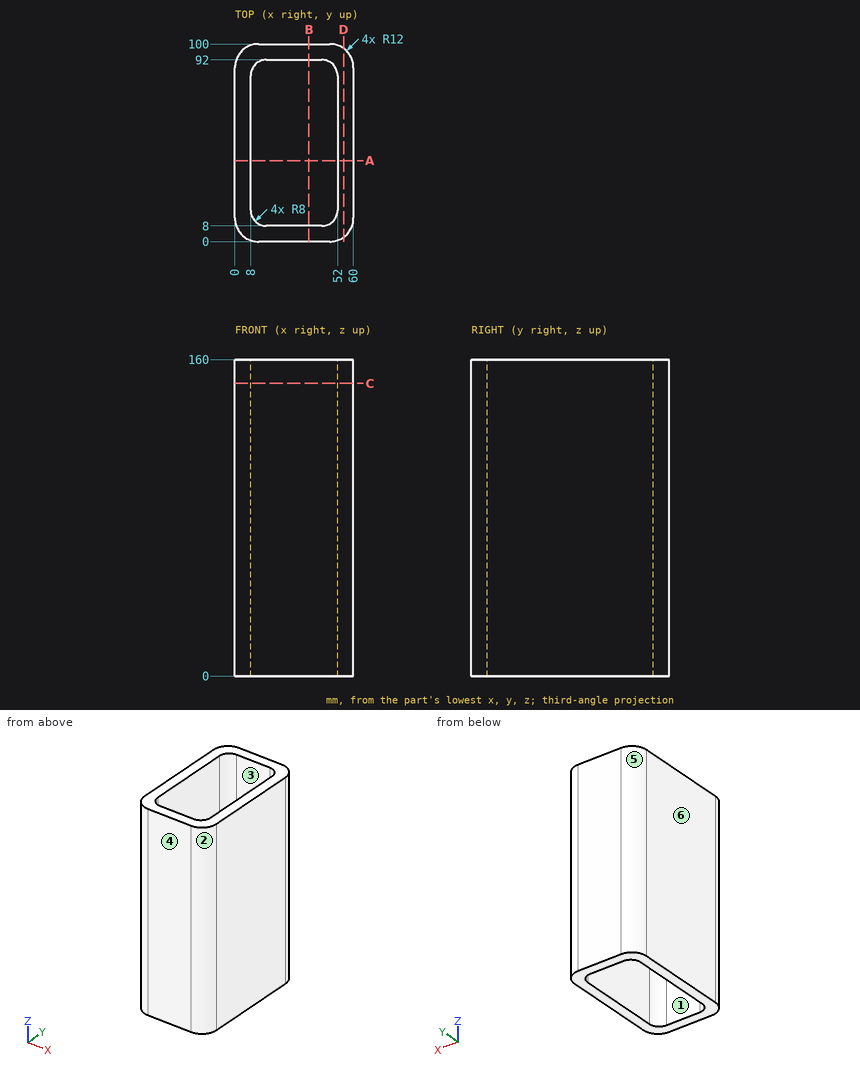
Geometry: see drawing. Coordinates: mm, zero at the bounding-box minimum. A direction names the side the tool comes from. Coordinates: 2 decimals unless noted, no trailing zeros. Loops run counter-clockwise (first coordinate to the right, second up) from the corner with the lowest first, then second, coordinate; pieces in that order, holes last. Notation, with made-up numbers: (-16, 68.5) -> (27, 68.5) arc R10 cw to (27, 80.5) -> close; hole circle Ø2 at (0, 26.5). An arc over 180 degrees is marked (long way). Write item = value, one per line. Start each with the question number.
Item 1: Reachability of the marked faces 1 and 2 from +Z, -Z, +X, -X, +Y, -Y: full face, straight path, thin tool, end or side. Return the list, or none.
Item 2: Material intervals for line 1 (X direction, y = 19.5, z = 152); line 2 (Y direction, x = 24, z = 7); line 3 (X direction, y = 9, z = 23.5), sorted ascending.
Item 3: Cut plane A-A, the plane y = 41. Return loops of the section in (x, z).
Item 4: Cut plane C-C, the plane z = 148. Return loops of the section in (x, y), plus the area to 3 significant figures.
Item 5: Mould query, pull axis Y, two halves, no side actions, for the marked faces 3, 4, 5 and 6. Classes: pulls with the +Y half, pulls with the -Y half, needs draft (parallel to the pull), parting line crosses it, or undercut.
Item 6: Cut plane B-B, the plane x = 37.5. Return loops of the section in (y, z).
Item 7: Cut plane D-D, the plane x = 55. Return loops of the section in (y, z), plus the area to 3 significant figures.
Ans:
q1.face_1 = +Z, -Z
q1.face_2 = +Z, -Z, +X, -Y
q2.line_1 = 0 to 8, 52 to 60
q2.line_2 = 0 to 8, 92 to 100
q2.line_3 = 0.38 to 12.13, 47.87 to 59.62
q3.outline = (0, 0) -> (8, 0) -> (8, 160) -> (0, 160) -> close; (52, 0) -> (60, 0) -> (60, 160) -> (52, 160) -> close
q4.outline = (0, 12) arc R12 ccw to (12, 0) -> (48, 0) arc R12 ccw to (60, 12) -> (60, 88) arc R12 ccw to (48, 100) -> (12, 100) arc R12 ccw to (0, 88) -> close; hole (8, 16) arc R8 ccw to (16, 8) -> (44, 8) arc R8 ccw to (52, 16) -> (52, 84) arc R8 ccw to (44, 92) -> (16, 92) arc R8 ccw to (8, 84) -> close
q4.area = 2,240 mm²
q5.face_3 = undercut
q5.face_4 = pulls with the -Y half
q5.face_5 = pulls with the +Y half
q5.face_6 = needs draft
q6.outline = (0, 0) -> (8, 0) -> (8, 160) -> (0, 160) -> close; (92, 0) -> (100, 0) -> (100, 160) -> (92, 160) -> close
q7.outline = (2.25, 0) -> (97.75, 0) -> (97.75, 160) -> (2.25, 160) -> close
q7.area = 15,300 mm²
